Work out the finished part from the listing and answer in its coordinate system (mm). Round coordinates to 2 decimals unless told otherwise and drop trailing zeros. Order: outer loops, then holes, each group sorted by start corner. A loop starts at its lowest first (then second) coordinate and runs counter-clockwise, first axis right, second up. Notation, with made-up numbers: M 32.25,32 L 63.25,32 A17 ccw 63.25,44 Z; hole C 9.5,-30.75 d3. An arc over 180 degrees is marked long. Answer as a JSON object with one key per item and string values. Group by question number.
Autodesk Inventor part; units mm, degrees
ref_plane "YZ Plane" through (0, 0, 0) normal (1, 0, 0) x (0, 1, 0)
ref_plane "XZ Plane" through (0, 0, 0) normal (0, 1, 0) x (-1, 0, 0)
ref_plane "XY Plane" through (0, 0, 0) normal (0, 0, 1) x (1, 0, 0)
sketch "Sketch1" plane through (0, 0, 0) normal (0, 0, 1) x (1, 0, 0)
  line L0 (0, 0) -> (0, 20)
  line L1 (20, 40) -> (40, 40)
  arc A0 (20, 40) -> (0, 20) centre (20, 20) ccw
  point P0 (0, 40)
  dimension "d0" = 40
  dimension "d1" = 40
  dimension "d2" = 20
sketch "Sketch2" plane through (0, 0, 0) normal (0, 1, 0) x (-1, 0, 0)
  circle A0 centre (0, 0) radius 19.5
  circle A1 centre (0, 0) radius 19.25
  dimension "d3" = 39
  dimension "d4" = 38.5
sweep "Sweep1" add profiles "Sketch2" path "Sketch1"
sketch "Sketch4" plane through (0, 0, 0) normal (0, 0, 1) x (1, 0, 0)
  circle A0 centre (0, 35.2694) radius 7.45
  point P0 (0, 0)
  dimension "d10" = 14.9
extrude "Extrusion2" cut sketch "Sketch4" against normal mid plane 40
properties part number "elbow"
Item 1: Consider L1, parallel to Z at x = 0, y = 14; L2, parallel to Z at x = 13.5, y = 13.5; L3, parallel to Y at x = 23, z = 15. Determine where each line is inside the solid, lowest interval first.
Item 2: Find section B-B (y = 15). Give the vertices of the cut face in (x, z).
Item 3: Each of these flat-tipped pins is pushed along its axis until it touches: pin 1 (6 mm diameter, centred on x = 21.5, y = 47, fed in from +Z); pin 2 (4 mm diameter, centred on x = 5.5, z = -10.5, fed in from -Y); pin 3 (8 mm diameter, centred on x = 10, z = 5.5, fed in from +Y). Where does it stop, or does it pass through?
Item 4: Find section C-C (x = 22.5). Give the vertices of the cut face in (y, z), and give its area (3 significant figures).
Item 5: Find section A-A (z = 0). Give the vertices of the cut face in (x, y).
Item 6: The mould has two halves that part along Z. Classify faces 1 (the cylindrical face through (30.14, 58.36, 5.78)), 2 (the cylindrical face through (30.14, 20.52, 0.86)): +Z half, -Z half, draft (parallel to the pull), parting line (faces both ways), or undercut.
Responses:
{
 "1": {"L1": "z = -19.5 to -19.25, 19.25 to 19.5", "L2": "z = -14.07 to -13.72, 13.72 to 14.07", "L3": "y = 27.54 to 27.94, 52.06 to 52.46"},
 "2": {"outline": "C 0,0 d39; hole C 0,0 d38.5"},
 "3": {"pin 1": "stops at z = 19.09", "pin 2": "stops at y = 51.23", "pin 3": "stops at y = 58.66"},
 "4": {"outline": "C 40,0 d39; hole C 40,0 d38.5", "area": "30.4 mm^2"},
 "5": {"outline": "M -19.5,0 L -19.25,0 L -19.25,20 A39.25 cw 20,59.25 L 40,59.25 L 40,59.5 L 20,59.5 A39.5 ccw -19.5,20 Z; M 19.25,0 L 19.5,0 L 19.5,20 A0.5 cw 20,20.5 L 40,20.5 L 40,20.75 L 20,20.75 A0.75 ccw 19.25,20 Z"},
 "6": {"face 1": "undercut", "face 2": "parting line"}
}
